For this review, take the finished solid that the model builds, in its own axes (mm). A direction names the side the tool comes from. Round coordinates to 2 decimals unless told otherwise and drop trailing zeros. Write each loop counter-clockwise with the first axis right and the second up, starting at its lowest first coordinate (ties: lowest second). Pieces come first, ordered by that corner, then holes. Notation, with made-up numbers: (-4.75, 13.5) -> (40.25, 13.5) arc R21 ccw to (40.25, 31.5) -> close; hole circle Ø2 at (66.5, 23.5). An arc over 180 degrees is marked (long way). Write each question's results on one line, items separated by ' | '. Start each with the question number.
Item 1: The part is to be moulded in two halves that separate along Z. For faces 1 (the flat face through (-54.86, 1.014, -85.804)), 2 (the flat face through (-1, 2, -1)), 3 (the flat face through (40.07, 0.986, -120.874)), say which applies: +Z half, -Z half, draft (parallel to the pull), parting line (faces both ways), or undercut.
Item 2: Add section D-D (y = 0.4). Count the separate pieces of the cut face and the enclosed holes in it, plus the area to 3 significant figures.
Item 3: To check wall thickness, follow line 1 along X through (y, z) = (0.8, -41.5); line 2 along X through (y, z) = (1.6, 15.25); line 3 along X through (y, z) = (1, 30). State the ranges of each line that lie inside material, in increasing order.
Item 4: Clearance check with flat-ended pins moving along their axes: pin 1 (1 mm diameter, centred on y = 1, z = 57, fed in from +X); pin 2 (1 mm diameter, centred on x = 57, y = 1.5, fed in from -Z); pin 3 (1 mm diameter, centred on y = 1.5, z = -84.5, fed in from +X). State where each tip first meets the part, or that it passes through.
Item 5: Tool access review of faces 4 (the flat face through (-101.425, 0.986, -107.346)), 5 (the flat face through (-101.51, 0.99, 146.58)), 6 (the flat face through (101.51, 0.99, -146.58)): name each direction out of +Z, -Z, +X, -X, +Y, -Y from which nothing blocks a thin tool from reaching the whole face with its end or side.
Item 6: Add section C-C (x = -61). State the section outline as (y, z) points.
Item 7: Add section B-B (x = -128). State the section outline as (y, z) points.
Item 8: Add section A-A (z = 22.5). State the section outline as (x, y) points, plus the area to 3 significant figures.
from build123d import *

# Parameters (mm, degrees)
Y_KSEKLIK_EKSTR_ZYON2_DEPTH = 2
IZIM3_R                     = 1.55
KES_EKSTR_ZYON1_DEPTH       = 2
KES_EKSTR_ZYON2_DEPTH       = 2
KES_EKSTR_ZYON3_DEPTH       = 20
PAH1_SIZE                   = 6
IZIM6_R                     = 2.5
KES_EKSTR_ZYON4_DEPTH       = 20
IZIM7_R                     = 1.55
KES_EKSTR_ZYON6_DEPTH       = 20
IZIM8_R                     = 1.55
KES_EKSTR_ZYON7_DEPTH       = 2
KES_EKSTR_ZYON8_DEPTH       = 10
IZIM10_R                    = 2.5
KES_EKSTR_ZYON9_DEPTH       = 10


with BuildPart() as part:
    # Çizim2 → Yükseklik-Ekstrüzyon2 (new body)
    with BuildSketch(Plane(origin=(0, 0, 0), x_dir=(1, 0, 0), z_dir=(0, 1, 0))):
        Polygon((-160.888072602, 157.241638979), (-45, 60), (-45, -60), (-160.888072602, -157.241638979), (-141.604444312, -180.222972272), (-65, -115.944211304), (-45, -115.944211304), (-35, -125.944211304), (35, -125.944211304), (45, -115.944211304), (65, -115.944211304), (141.604444312, -180.222972272), (160.888072602, -157.241638979), (45, -60), (45, 60), (160.888072602, 157.241638979), (141.604444312, 180.222972272), (65, 115.944211304), (45, 115.944211304), (35, 125.944211304), (-35, 125.944211304), (-45, 115.944211304), (-65, 115.944211304), (-141.604444312, 180.222972272), align=None)
    extrude(amount=Y_KSEKLIK_EKSTR_ZYON2_DEPTH)

    # Çizim3 → Kes-Ekstrüzyon1 (cut)
    with BuildSketch(Plane(origin=(0, 2, 0), x_dir=(1, 0, 0), z_dir=(0, 1, 0))):
        with Locations(Location((-22.5, 90.944211304, 0), (0, 0, 270))):
            Circle(IZIM3_R)
        with Locations(Location((22.5, 90.944211304, 0), (0, 0, 270))):
            Circle(IZIM3_R)
        with Locations(Location((-22.5, 45.944211304, 0), (0, 0, 270))):
            Circle(IZIM3_R)
        with Locations(Location((22.5, 45.944211304, 0), (0, 0, 270))):
            Circle(IZIM3_R)
        with Locations(Location((-15.25, 15.25, 0), (0, 0, 270))):
            Circle(IZIM3_R)
        with Locations(Location((15.25, 15.25, 0), (0, 0, 270))):
            Circle(IZIM3_R)
        with Locations(Location((15.25, -15.25, 0), (0, 0, 270))):
            Circle(IZIM3_R)
        with Locations(Location((-15.25, -15.25, 0), (0, 0, 270))):
            Circle(IZIM3_R)
    extrude(amount=-KES_EKSTR_ZYON1_DEPTH, mode=Mode.SUBTRACT)

    # Çizim4 → Kes-Ekstrüzyon2 (cut)
    with BuildSketch(Plane(origin=(0, 2, 0), x_dir=(1, 0, 0), z_dir=(0, 1, 0))):
        Polygon((-2.5, -111.614084285), (0, -115.944211304), (2.5, -111.614084285), align=None)
    extrude(amount=-KES_EKSTR_ZYON2_DEPTH, mode=Mode.SUBTRACT)

    # Çizim5 → Kes-Ekstrüzyon3 (cut)
    with BuildSketch(Plane(origin=(0, 2, 0), x_dir=(1, 0, 0), z_dir=(0, 1, 0))):
        Polygon((-65, 95.944211304), (-45, 95.944211304), (-45, 75.944211304), align=None)
        Polygon((45, 75.944211304), (65, 95.944211304), (45, 95.944211304), align=None)
        Polygon((65, -95.944211304), (45, -95.944211304), (45, -75.944211304), align=None)
        Polygon((-45, -75.944211304), (-65, -95.944211304), (-45, -95.944211304), align=None)
    extrude(amount=-KES_EKSTR_ZYON3_DEPTH, mode=Mode.SUBTRACT)

    # Pah1
    pah1_edges = [part.edges().sort_by_distance(p)[0] for p in [
        (-160.888072602, 1, -157.241638979),
        (-141.604444312, 1, -180.222972272),
        (141.604444312, 1, -180.222972272),
        (160.888072602, 1, -157.241638979),
        (160.888072602, 1, 157.241638979),
        (141.604444312, 1, 180.222972272),
        (-141.604444312, 1, 180.222972272),
        (-160.888072602, 1, 157.241638979),
    ]]
    chamfer(pah1_edges, length=PAH1_SIZE)

    # Çizim6 → Kes-Ekstrüzyon4 (cut)
    with BuildSketch(Plane(origin=(0, 2, 0), x_dir=(1, 0, 0), z_dir=(0, 1, 0))):
        with Locations(Location((-139.75559181, 159.09049148, 0), (0, 0, 270))):
            Circle(IZIM6_R)
        with Locations(Location((-101.453369654, 126.951110996, 0), (0, 0, 270))):
            Circle(IZIM6_R)
        with Locations(Location((139.75559181, 159.09049148, 0), (0, 0, 270))):
            Circle(IZIM6_R)
        with Locations(Location((101.453369654, 126.951110996, 0), (0, 0, 270))):
            Circle(IZIM6_R)
        with Locations(Location((-139.75559181, -159.09049148, 0), (0, 0, 270))):
            Circle(IZIM6_R)
        with Locations(Location((-101.453369654, -126.951110996, 0), (0, 0, 270))):
            Circle(IZIM6_R)
        with Locations(Location((101.453369654, -126.951110996, 0), (0, 0, 270))):
            Circle(IZIM6_R)
        with Locations(Location((139.75559181, -159.09049148, 0), (0, 0, 270))):
            Circle(IZIM6_R)
    extrude(amount=-KES_EKSTR_ZYON4_DEPTH, mode=Mode.SUBTRACT)

    # Çizim7 → Kes-Ekstrüzyon6 (cut)
    with BuildSketch(Plane(origin=(0, 2, 0), x_dir=(1, 0, 0), z_dir=(0, 1, 0))):
        with Locations(Location((-24.5, -44.444211304, 0), (0, 0, 270))):
            Circle(IZIM7_R)
        with Locations(Location((-24.5, -102.444211304, 0), (0, 0, 270))):
            Circle(IZIM7_R)
        with Locations(Location((24.5, -102.444211304, 0), (0, 0, 270))):
            Circle(IZIM7_R)
        with Locations(Location((24.5, -44.444211304, 0), (0, 0, 270))):
            Circle(IZIM7_R)
    extrude(amount=-KES_EKSTR_ZYON6_DEPTH, mode=Mode.SUBTRACT)

    # Çizim8 → Kes-Ekstrüzyon7 (cut)
    with BuildSketch(Plane(origin=(0, 2, 0), x_dir=(1, 0, 0), z_dir=(0, 1, 0))):
        with Locations(Location((0, 69.944211304, 0), (0, 0, 270))):
            Circle(IZIM8_R)
        with Locations(Location((-21.75, 100.944211304, 0), (0, 0, 270))):
            Circle(IZIM8_R)
        with Locations(Location((21.75, 100.944211304, 0), (0, 0, 270))):
            Circle(IZIM8_R)
    extrude(amount=-KES_EKSTR_ZYON7_DEPTH, mode=Mode.SUBTRACT)

    # Çizim9 → Kes-Ekstrüzyon8 (cut)
    with BuildSketch(Plane(origin=(0, 2, 0), x_dir=(1, 0, 0), z_dir=(0, 1, 0))):
        with BuildLine():
            Line((-35, 50), (-35, -50))
            ThreePointArc((-35, -50), (-37.5, -52.5), (-40, -50))
            Line((-40, -50), (-40, 50))
            ThreePointArc((-40, 50), (-37.5, 52.5), (-35, 50))
        make_face()
        with BuildLine():
            Line((40, 50), (40, -50))
            ThreePointArc((40, -50), (37.5, -52.5), (35, -50))
            Line((35, -50), (35, 50))
            ThreePointArc((35, 50), (37.5, 52.5), (40, 50))
        make_face()
    extrude(amount=-KES_EKSTR_ZYON8_DEPTH, mode=Mode.SUBTRACT)

    # Çizim10 → Kes-Ekstrüzyon9 (cut)
    with BuildSketch(Plane(origin=(0, 2, 0), x_dir=(1, 0, 0), z_dir=(0, 1, 0))):
        with Locations(Location((25.75, -30, 0), (0, 0, 270))):
            Circle(IZIM10_R)
        with Locations(Location((-25.75, -30, 0), (0, 0, 270))):
            Circle(IZIM10_R)
        with Locations(Location((25.75, 30, 0), (0, 0, 270))):
            Circle(IZIM10_R)
        with Locations(Location((-25.75, 30, 0), (0, 0, 270))):
            Circle(IZIM10_R)
    extrude(amount=-KES_EKSTR_ZYON9_DEPTH, mode=Mode.SUBTRACT)


solid = part.part
Responses:
1) face 1: undercut | face 2: draft | face 3: -Z half
2) separate pieces: 1 | enclosed holes: 34 | area: 37,400 mm^2
3) line 1: x = -45 to -40, -35 to 35, 40 to 45 | line 2: x = -45 to -40, -35 to -16.8, -13.7 to 13.7, 16.8 to 35, 40 to 45 | line 3: x = -45 to -40, -35 to -28.25, -23.25 to 23.25, 28.25 to 35, 40 to 45
4) pin 1: stops at x = 45 | pin 2: stops at z = -115.94 | pin 3: stops at x = 74.79
5) face 4: -X, +Y, -Y | face 5: +Z, +Y, -Y | face 6: -Z, +Y, -Y
6) outline: (0, -115.94) -> (2, -115.94) -> (2, -95.94) -> (0, -95.94) -> close; (0, -91.94) -> (2, -91.94) -> (2, -73.43) -> (0, -73.43) -> close; (0, 73.43) -> (2, 73.43) -> (2, 91.94) -> (0, 91.94) -> close; (0, 95.94) -> (2, 95.94) -> (2, 115.94) -> (0, 115.94) -> close
7) outline: (0, -168.81) -> (2, -168.81) -> (2, -129.65) -> (0, -129.65) -> close; (0, 129.65) -> (2, 129.65) -> (2, 168.81) -> (0, 168.81) -> close
8) outline: (-45, 0) -> (-40, 0) -> (-40, 2) -> (-45, 2) -> close; (-35, 0) -> (35, 0) -> (35, 2) -> (-35, 2) -> close; (40, 0) -> (45, 0) -> (45, 2) -> (40, 2) -> close | area: 160 mm^2
